Read the model definition and answer for the solid it produces. Units are mm, in the model's axes. Coordinates: 2 decimals unless noted, no trailing zeros. Loops run counter-clockwise (first coordinate to the right, second up) from the corner with the lowest first, then second, coordinate; pieces in that order, holes last. Notation, with made-up numbers: (17, 10) -> (48, 10) arc R24 ccw to (48, 30) -> close; hole circle Ø5 at (13, 7). An arc over 180 degrees is marked (long way). Answer as a JSON object with one key per item and string values. Group by question number.
1) Flat-ended cylindrical pins translate along their axes: P1, Ø1.5, axis at x = -36.5, z = 4, coming from the -Y side; P2, Ø2.5, axis at y = 9.5, z = 3, coming from the -X side. Find the tip coordinate at first contact, or state that the pin passes through.
2) Consider probe 1 along Y at (x, z) = (-36.5, 0.3); probe 2 along Y at (x, z) = (-31.5, 0.8); probe 3 along X at (y, z) = (101, 1.5). Determine where each line is inside the solid, lowest interval first. Write a range as [from, to].
3) Section C-C, the plane y = 89.5 is taken. Give the vertices of the cut face in (x, z), plus the area to 3 significant figures.
4) Section D-D, the plane x = -18.5 is taken. Give the vertices of the cut face in (y, z).
5) Section A-A, the plane x = -36.83 is taken. Give the vertices of the cut face in (y, z), plus the area to 3 significant figures.
6) Section B-B, the plane z = 0.85 is taken. Count the separate pieces of the cut face and the enclosed holes in it, plus the area to 3 significant figures.
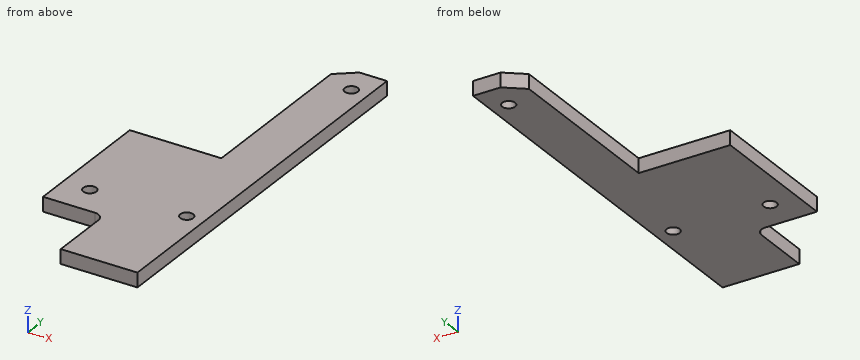
from build123d import *

# Parameters (mm, degrees)
BOSS_EXTRUDE1_DEPTH = 4.7625
SKETCH3_R           = 2.15265
CUT_EXTRUDE1_DEPTH  = 139.651562942


with BuildPart() as part:
    # Sketch1 → Boss-Extrude1 (new body)
    with BuildSketch(Plane.XY):
        with BuildLine():
            Line((-15.392138512, 125.820167161), (-15.392138512, 68.343175012))
            Line((-15.392138512, 68.343175012), (-45.72, 68.343175012))
            Line((-45.72, 68.343175012), (-45.72, 22.86))
            Line((-45.72, 22.86), (-28.575, 22.86))
            ThreePointArc((-28.575, 22.86), (-26.32993597, 21.93006403), (-25.4, 19.685))
            Line((-25.4, 19.685), (-25.4, 0))
            Line((-25.4, 0), (0, 0))
            Line((0, 0), (0, 130.81))
            Line((0, 130.81), (-9.144, 130.81))
            Line((-9.144, 130.81), (-15.392138512, 125.820167161))
        make_face()
    extrude(amount=BOSS_EXTRUDE1_DEPTH)

    # Sketch3 → Cut-Extrude1 (cut, through all)
    with BuildSketch(Plane(origin=(0, 0, 0), x_dir=(-1, 0, 0), z_dir=(0, 0, -1))):
        with Locations((5.715, 121.158)):
            Circle(SKETCH3_R)
        with Locations((5.715, 34.925)):
            Circle(SKETCH3_R)
        with Locations((36.83, 33.3375)):
            Circle(SKETCH3_R)
    extrude(amount=-CUT_EXTRUDE1_DEPTH, mode=Mode.SUBTRACT)


solid = part.part
Determined:
{
 "1": {"P1": "y = 22.86", "P2": "x = -25.4"},
 "2": {"probe 1": "[22.86, 31.21], [35.46, 68.34]", "probe 2": "[22.86, 68.34]", "probe 3": "[-15.39, 0]"},
 "3": {"outline": "(-15.39, 0) -> (0, 0) -> (0, 4.76) -> (-15.39, 4.76) -> close", "area": "73.3 mm²"},
 "4": {"outline": "(0, 0) -> (68.34, 0) -> (68.34, 4.76) -> (0, 4.76) -> close"},
 "5": {"outline": "(22.86, 0) -> (31.18, 0) -> (31.18, 4.76) -> (22.86, 4.76) -> close; (35.49, 0) -> (68.34, 0) -> (68.34, 4.76) -> (35.49, 4.76) -> close", "area": "196 mm²"},
 "6": {"separate pieces": "1", "enclosed holes": "3", "area": "3,560 mm²"}
}
